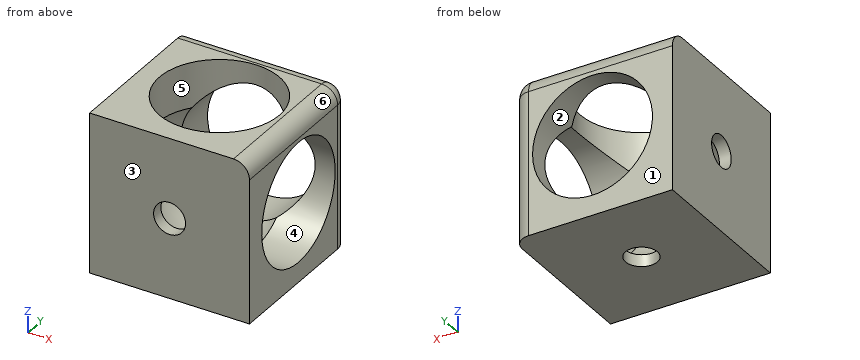
from build123d import *

# Parameters (mm, degrees)
SKETCH1_W           = 40
SKETCH1_H           = 40
BOSS_EXTRUDE1_DEPTH = 20
FILLET1_R           = 4
SKETCH12_R          = 15
CUT_EXTRUDE2_DEPTH  = 20
SKETCH13_R          = 15
CUT_EXTRUDE3_DEPTH  = 20
SKETCH14_R          = 15
CUT_EXTRUDE4_DEPTH  = 20
SKETCH15_R          = 4
CUT_EXTRUDE5_DEPTH  = 20
SKETCH16_R          = 4
CUT_EXTRUDE6_DEPTH  = 20
SKETCH17_R          = 4
CUT_EXTRUDE7_DEPTH  = 20


with BuildPart() as part:
    # Sketch1 → Boss-Extrude1 (new body, symmetric)
    with BuildSketch(Plane(origin=(0, 0, 0), x_dir=(1, 0, 0), z_dir=(0, 1, 0))):
        Rectangle(SKETCH1_W, SKETCH1_H)
    extrude(amount=BOSS_EXTRUDE1_DEPTH, both=True)

    # Fillet1
    fillet1_edges = [part.edges().sort_by_distance(p)[0] for p in [
        (20, 20, 0),
        (20, 0, 20),
        (0, 20, 20),
    ]]
    fillet(fillet1_edges, radius=FILLET1_R)

    # Sketch2 → Cut-Revolve1 (revolve, cut)
    with BuildSketch(Plane(origin=(0, 0, 0), x_dir=(1, 0, 0), z_dir=(0, 1, 0))):
        with BuildLine():
            Line((0, 17.5), (0, -17.5))
            ThreePointArc((0, -17.5), (-17.5, 0), (0, 17.5))
        make_face()
    revolve(axis=Axis((0, 0, -20.989422068), (0, 0, 1)), mode=Mode.SUBTRACT)

    # Sketch12 → Cut-Extrude2 (cut)
    with BuildSketch(Plane(origin=(0, 20, 0), x_dir=(1, 0, 0), z_dir=(0, 1, 0))):
        Circle(SKETCH12_R)
    extrude(amount=-CUT_EXTRUDE2_DEPTH, mode=Mode.SUBTRACT)

    # Sketch13 → Cut-Extrude3 (cut)
    with BuildSketch(Plane(origin=(20, 0, 0), x_dir=(0, 0, -1), z_dir=(1, 0, 0))):
        Circle(SKETCH13_R)
    extrude(amount=-CUT_EXTRUDE3_DEPTH, mode=Mode.SUBTRACT)

    # Sketch14 → Cut-Extrude4 (cut)
    with BuildSketch(Plane.XY.offset(20)):
        with Locations((0, 0.367598837)):
            Circle(SKETCH14_R)
    extrude(amount=-CUT_EXTRUDE4_DEPTH, mode=Mode.SUBTRACT)

    # Sketch15 → Cut-Extrude5 (cut)
    with BuildSketch(Plane(origin=(0, 0, -20), x_dir=(-1, 0, 0), z_dir=(0, 0, -1))):
        Circle(SKETCH15_R)
    extrude(amount=-CUT_EXTRUDE5_DEPTH, mode=Mode.SUBTRACT)

    # Sketch16 → Cut-Extrude6 (cut)
    with BuildSketch(Plane.XZ.offset(20)):
        Circle(SKETCH16_R)
    extrude(amount=-CUT_EXTRUDE6_DEPTH, mode=Mode.SUBTRACT)

    # Sketch17 → Cut-Extrude7 (cut)
    with BuildSketch(Plane.ZY.offset(20)):
        Circle(SKETCH17_R)
    extrude(amount=-CUT_EXTRUDE7_DEPTH, mode=Mode.SUBTRACT)


solid = part.part
Here's how the part is built. I have some questions about the finished solid (model axes, mm). Face numbers are marked on the shaded views. A direction names the side the tool comes from. Give positions to 0.01 mm unless a question says otherwise; leave off trailing zeros. Loops run counter-clockwise (first coordinate to the right, second up) from the corner with the lowest first, then second, coordinate; pieces in that order, holes last. Notation, with made-up numbers: (80, 66) -> (100, 66) arc R8 cw to (100, 77) -> close; hole circle Ø6 at (39, 45). An arc over 180 degrees is marked (long way). One line per item, written item: value.
Q1. I'm going to push flat-ended pins straight in: pin 1 Ø24 at (x, y) = (0, 0.37) entering from +Z; pin 2 Ø1 at (y, z) = (-13.5, -5) entering from +X; pin 3 Ø2 at (x, y) = (-1, -9.5) entering from +Z; pin 4 Ø24 at (x, z) = (0, 0) entering from -Y. Where does each tip first touch, or does it pass through?
Answers follow:
pin 1: z = -12.48
pin 2: x = -9.18
pin 3: z = -13.96
pin 4: y = -20
Q2. We'd pull the mould along Y, two halves only. Please class the marked faces 3, 4, 5 and 6: pulls with the +Y half, pulls with the -Y half, needs draft (parallel to the pull), parting line crosses it, or undercut.
Answers follow:
face 3: pulls with the -Y half
face 4: undercut
face 5: undercut
face 6: needs draft
Q3. Suppose I cut it at B-B on x = 0. Please give me the cut outline in (y, z).
Answers follow:
outline: (-20, -20) -> (-4, -20) -> (-4, -17.04) arc R17.5 cw to (-17.04, -4) -> (-20, -4) -> close; (-20, 4) -> (-17.04, 4) arc R17.5 cw to (-14.63, 9.6) -> (-14.63, 20) -> (-20, 20) -> close; (4, -20) -> (20, -20) -> (20, -15) -> (9.01, -15) arc R17.5 cw to (4, -17.04) -> close; (15.37, 15) -> (20, 15) -> (20, 16) arc R4 ccw to (16, 20) -> (15.37, 20) -> close
Q4. Suppose I cut it at C-C on z = -9. Please give me the cut outline in (x, y).
Answers follow:
outline: (-20, -20) -> (20, -20) -> (20, -12) -> (9.01, -12) arc R15.01 cw to (-12, 9.01) -> (-12, 20) -> (-20, 20) -> close; (12, 12) -> (20, 12) -> (20, 16) arc R4 ccw to (16, 20) -> (12, 20) -> close
Q5. On a 3-axis mill with a long thin cutter (end or side, diameter ignored), from which of +Z, -Z, +X, -X, +Y, -Y can I reach the whole of each face in a straight line? I mean the marked faces 1 and 2. Say none if no direction works.
Answers follow:
face 1: +Z, -Z, +X, -X, +Y
face 2: +Y
Q6. Suppose I cut it at D-D on x = -8. Please give me the cut outline in (y, z), then the cut area to 3 significant figures.
Answers follow:
outline: (-20, -20) -> (20, -20) -> (20, -12.69) -> (9.01, -12.69) arc R15.56 cw to (-12.32, 9.51) -> (-12.32, 20) -> (-20, 20) -> close; (13.06, 12.69) -> (20, 12.69) -> (20, 16) arc R4 ccw to (16, 20) -> (13.06, 20) -> close
area: 518 mm^2
Q7. Suppose I cut it at A-A on z = 0. Please give me the cut outline in (x, y).
Answers follow:
outline: (-20, -20) -> (-4, -20) -> (-4, -17.04) arc R17.5 cw to (-17.04, -4) -> (-20, -4) -> close; (-20, 4) -> (-17.04, 4) arc R17.5 cw to (-15, 9.01) -> (-15, 20) -> (-20, 20) -> close; (4, -20) -> (20, -20) -> (20, -15) -> (9.01, -15) arc R17.5 cw to (4, -17.04) -> close; (15, 15) -> (20, 15) -> (20, 16) arc R4 ccw to (16, 20) -> (15, 20) -> close
Q8. If I drill on line 1 along Z through (x, y) = (0, -18); line 2 along Y through (x, z) = (0, 16), over which ranges is the centre line in solid material (lowest first)?
Answers follow:
line 1: -20 to -4, 4 to 20
line 2: -20 to -14.63, 15.37 to 20
